Study the drawing (mm; zero at the part's minimum x, y, z) and answer. Coordinates: 2 decimals unless noted, no trailing zeros. Order: outer loops, then holes, each group sorted by start corner. A loop starts at its lowest first (then second) coordinate and runs counter-clockwise, first axis right, second up. Notation, with made-up numbers: M -6,-9.5 L 35,-9.5 A22 cw 35,23.5 Z; hole C -33,15.25 d8. An arc over 180 degrees is marked long. Use a Markdown table: item, result. Add a question column.
1) Find section D-D on y = 36. Write down the section's boundary in (x, z), plus the area to 3 significant figures.
2) Find section C-C on x = 11. Write down the section's boundary in (y, z), plus the area to 3 significant figures.
3) Find section A-A on y = 11. Write down the section's boundary in (x, z), plus the area to 3 significant figures.
4) Find section B-B on z = 17. Write down the section's boundary in (x, y).
5) This flat-tipped pin is pushed along its axis until it touches: pin 1 Ø5 at (x, y) = (48, 20) entering from -Z. Where does it stop, or does it pass through?
6) Find the intervals of material crossed by probe 1 along X at (y, z) = (11, 15); probe 2 along Y at (x, z) = (11, 8); probe 3 along Y at (x, z) = (59, 19), in increasing order. Write a range as [from, to].
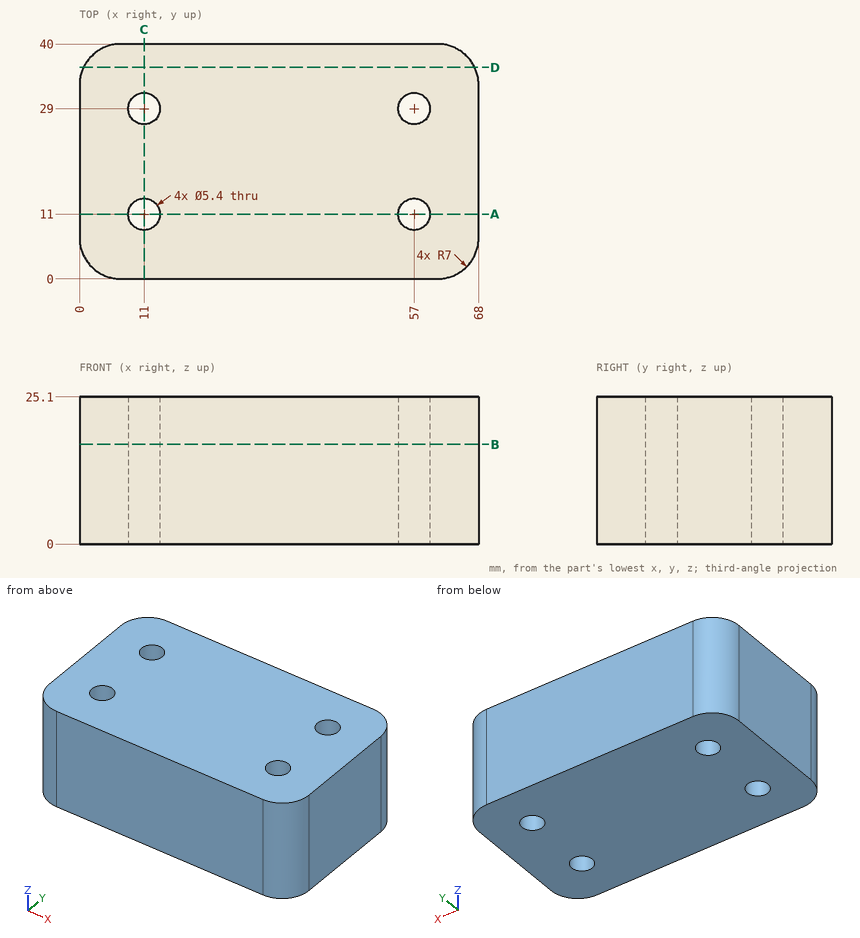
Check result:
| question | item | result |
|---|---|---|
| 1 | outline | M 0.68,0 L 67.32,0 L 67.32,25.1 L 0.68,25.1 Z |
| 1 | area | 1,670 mm2 |
| 2 | outline | M 0,0 L 8.3,0 L 8.3,25.1 L 0,25.1 Z; M 13.7,0 L 26.3,0 L 26.3,25.1 L 13.7,25.1 Z; M 31.7,0 L 40,0 L 40,25.1 L 31.7,25.1 Z |
| 2 | area | 733 mm2 |
| 3 | outline | M 0,0 L 8.3,0 L 8.3,25.1 L 0,25.1 Z; M 13.7,0 L 54.3,0 L 54.3,25.1 L 13.7,25.1 Z; M 59.7,0 L 68,0 L 68,25.1 L 59.7,25.1 Z |
| 3 | area | 1,440 mm2 |
| 4 | outline | M 0,7 A7 ccw 7,0 L 61,0 A7 ccw 68,7 L 68,33 A7 ccw 61,40 L 7,40 A7 ccw 0,33 Z; hole C 11,11 d5.4; hole C 11,29 d5.4; hole C 57,11 d5.4; hole C 57,29 d5.4 |
| 5 | pin 1 | stops at z = 0 |
| 6 | probe 1 | x = [0, 8.3], [13.7, 54.3], [59.7, 68] |
| 6 | probe 2 | y = [0, 8.3], [13.7, 26.3], [31.7, 40] |
| 6 | probe 3 | y = [0, 9.19], [12.81, 27.19], [30.81, 40] |
